from build123d import *

# Parameters (mm, degrees)
F1_DEPTH = 6.35
F2_DEPTH = 12.7


# Not quite as in the source:
# - a feature names something its author has since deleted; it is built from what else it names


with BuildPart() as f1:
    # F0 (on Top) → F1 (new body)
    with BuildSketch(Plane.XY):
        Polygon((1.6, 1.6), (27, 1.6), (27, 7.95), (7.95, 7.95), (-7.95, 7.95), (-7.95, -7.95), (-7.95, -27), (-1.6, -27), (-1.6, -1.6), (-1.6, 1.6), align=None)
        Polygon((27, -7.95), (27, -1.6), (1.6, -1.6), (1.6, -27), (7.95, -27), (7.95, -7.95), align=None)
        Polygon((27, 0), (27, 1.6), (1.6, 1.6), (-1.6, 1.6), (-1.6, -1.6), (-1.6, -27), (0, -27), (1.6, -27), (1.6, -1.6), (27, -1.6), align=None)
    extrude(amount=-F1_DEPTH)

    # F0 (on Top) → F2 (join)
    with BuildSketch(Plane.XY):
        Polygon((1.6, 1.6), (27, 1.6), (27, 7.95), (7.95, 7.95), (-7.95, 7.95), (-7.95, -7.95), (-7.95, -27), (-1.6, -27), (-1.6, -1.6), (-1.6, 1.6), align=None)
        Polygon((27, -7.95), (27, -1.6), (1.6, -1.6), (1.6, -27), (7.95, -27), (7.95, -7.95), align=None)
    extrude(amount=F2_DEPTH)


solid = f1.part
Geometry check sheet. Reference: the model listing, model coordinates, mm. A direction names the side the tool comes from. Round coordinates to 2 decimals unless told otherwise and drop trailing zeros. Order: outer loops, then holes, each group sorted by start corner. A loop starts at its lowest first (then second) coordinate and runs counter-clockwise, first axis right, second up. Notation, with made-up numbers: M -17,-1.5 L 38,-1.5 A4 ccw 38,3.5 Z; hole C -36,-31.75 d4. An arc over 180 degrees is marked long. Answer in a Markdown table with one row per item.
(1) Sectioned sample at A-A, the plane z = 10. Record the cut outline in (x, y).
Responses:
| item | result |
|---|---|
| outline | M -7.95,-27 L -1.6,-27 L -1.6,1.6 L 27,1.6 L 27,7.95 L -7.95,7.95 Z; M 1.6,-27 L 7.95,-27 L 7.95,-7.95 L 27,-7.95 L 27,-1.6 L 1.6,-1.6 Z |
(2) Draft check along X on faces 5 (the face through (10, 7.95, 3)), 6 (the face through (1.6, -14, 6)), 7 (the face through (-7.95, -9, 3)). Enter one of: released by +X, released by -X, zero draft, split by the parting line, or undercut.
Responses:
| item | result |
|---|---|
| face 5 | zero draft |
| face 6 | undercut |
| face 7 | released by -X |
(3) Sectioned sample at B-B, the plane x = 14. Record the cut outline in (y, z).
Responses:
| item | result |
|---|---|
| outline | M -7.95,-6.35 L 7.95,-6.35 L 7.95,12.7 L 1.6,12.7 L 1.6,0 L -1.6,0 L -1.6,12.7 L -7.95,12.7 Z |
(4) Sectioned sample at D-D, the plane z = -3.75. Record the cut outline in (x, y), and give its area (3 significant figures).
Responses:
| item | result |
|---|---|
| outline | M -7.95,-27 L 7.95,-27 L 7.95,-7.95 L 27,-7.95 L 27,7.95 L -7.95,7.95 Z |
| area | 859 mm² |
(5) Sectioned sample at C-C, the plane y = -5. Record the cut outline in (x, z).
Responses:
| item | result |
|---|---|
| outline | M -7.95,-6.35 L 27,-6.35 L 27,12.7 L 1.6,12.7 L 1.6,0 L -1.6,0 L -1.6,12.7 L -7.95,12.7 Z |
(6) Scan lines: probe 1 along X at (y, z) = (-5.5, 0.5); probe 2 along X at (y, z) = (-13, 7). Record each from-to range of solid material in increasing order. Write a range as from..to.
Responses:
| item | result |
|---|---|
| probe 1 | x = -7.95..-1.6, 1.6..27 |
| probe 2 | x = -7.95..-1.6, 1.6..7.95 |
(7) Tool access check on faces 1 (the face through (27, -2, 3)), 2 (the face through (-1.6, -13, 6)), 3 (the face through (14, -1.6, 6)), 4 (the face through (7.95, -18, 3)). Record the directions out of +Z, -Z, +X, -X, +Y, -Y that give a thin tool (end or side, any length) a straight path to the whole face; none if there is none.
Responses:
| item | result |
|---|---|
| face 1 | +Z, -Z, +X, +Y, -Y |
| face 2 | +Z, -Y |
| face 3 | +Z, +X |
| face 4 | +Z, -Z, +X, -Y |
(8) Go/stop test with flat-tipped pins: P1, Ø4, axis at x = 16, z = 4, coming from the -Y side; P2, Ø6, axis at y = -21, z = 8, coming from the +X side. Record where each tip stops, or that it passes through.
Responses:
| item | result |
|---|---|
| P1 | stops at y = -7.95 |
| P2 | stops at x = 7.95 |
